```python
from build123d import *

# Parameters (mm, degrees)
SALIENTE_EXTRUIR3_DEPTH = 47
CROQUIS4_W              = 1.5
CROQUIS4_H              = 87
SALIENTE_EXTRUIR4_DEPTH = 47
CROQUIS5_OUTSIDE_W      = 115.342
CROQUIS5_OUTSIDE_H      = 115.342
CROQUIS5_OUTSIDE_R      = 43.5
CORTAR_EXTRUIR1_DEPTH   = 47


with BuildPart() as part:
    # Croquis3 → Saliente-Extruir3 (new body)
    with BuildSketch(Plane(origin=(0, 0, 0), x_dir=(1, 0, 0), z_dir=(0, 1, 0))):
        with BuildLine():
            Line((-43.5, 1.25), (-12.939764295, 1.25))
            ThreePointArc((-12.939764295, 1.25), (0, 13), (12.939764295, 1.25))
            Line((12.939764295, 1.25), (43.5, 1.25))
            Line((43.5, 1.25), (43.5, -1.25))
            Line((43.5, -1.25), (12.939764295, -1.25))
            ThreePointArc((12.939764295, -1.25), (0, -13), (-12.939764295, -1.25))
            Line((-12.939764295, -1.25), (-43.5, -1.25))
            Line((-43.5, -1.25), (-43.5, 1.25))
        make_face()
    extrude(amount=SALIENTE_EXTRUIR3_DEPTH)

    # Croquis4 → Saliente-Extruir4 (add)
    with BuildSketch(Plane(origin=(0, 47, 0), x_dir=(1, 0, 0), z_dir=(0, 1, 0))):
        with Locations((-42.437546, 0)):
            Rectangle(CROQUIS4_W, CROQUIS4_H)
        with Locations((-38.395758095, 0)):
            Rectangle(CROQUIS4_W, CROQUIS4_H)
        with Locations((-34.35397019, 0)):
            Rectangle(CROQUIS4_W, CROQUIS4_H)
        with Locations((-30.312182286, 0)):
            Rectangle(CROQUIS4_W, CROQUIS4_H)
        with Locations((-26.270394381, 0)):
            Rectangle(CROQUIS4_W, CROQUIS4_H)
        with Locations((-22.228606476, 0)):
            Rectangle(CROQUIS4_W, CROQUIS4_H)
        with Locations((-18.186818571, 0)):
            Rectangle(CROQUIS4_W, CROQUIS4_H)
        with Locations((-14.145030667, 0)):
            Rectangle(CROQUIS4_W, CROQUIS4_H)
        with Locations((-10.103242762, 0)):
            Rectangle(CROQUIS4_W, CROQUIS4_H)
        with Locations((-6.061454857, 0)):
            Rectangle(CROQUIS4_W, CROQUIS4_H)
        with Locations((-2.019666952, 0)):
            Rectangle(CROQUIS4_W, CROQUIS4_H)
        with Locations((2.022120952, 0)):
            Rectangle(CROQUIS4_W, CROQUIS4_H)
        with Locations((6.063908857, 0)):
            Rectangle(CROQUIS4_W, CROQUIS4_H)
        with Locations((10.105696762, 0)):
            Rectangle(CROQUIS4_W, CROQUIS4_H)
        with Locations((14.147484667, 0)):
            Rectangle(CROQUIS4_W, CROQUIS4_H)
        with Locations((18.189272571, 0)):
            Rectangle(CROQUIS4_W, CROQUIS4_H)
        with Locations((22.231060476, 0)):
            Rectangle(CROQUIS4_W, CROQUIS4_H)
        with Locations((26.272848381, 0)):
            Rectangle(CROQUIS4_W, CROQUIS4_H)
        with Locations((30.314636286, 0)):
            Rectangle(CROQUIS4_W, CROQUIS4_H)
        with Locations((34.35642419, 0)):
            Rectangle(CROQUIS4_W, CROQUIS4_H)
        with Locations((38.398212095, 0)):
            Rectangle(CROQUIS4_W, CROQUIS4_H)
        with Locations((42.44, 0)):
            Rectangle(CROQUIS4_W, CROQUIS4_H)
    extrude(amount=-SALIENTE_EXTRUIR4_DEPTH)

    # Croquis5 outside → Cortar-Extruir1 (cut)
    with BuildSketch(Plane(origin=(0, 47, 0), x_dir=(1, 0, 0), z_dir=(0, 1, 0))):
        Rectangle(CROQUIS5_OUTSIDE_W, CROQUIS5_OUTSIDE_H)
        Circle(CROQUIS5_OUTSIDE_R, mode=Mode.SUBTRACT)
    extrude(amount=-CORTAR_EXTRUIR1_DEPTH, mode=Mode.SUBTRACT)


solid = part.part
```
Model file for the job. Use its own axes, mm. A direction names the side the tool comes from. Round coordinates to 2 decimals unless told otherwise and drop trailing zeros. Write each loop counter-clockwise with the first axis right and the second up, starting at its lowest first coordinate (ties: lowest second). Pieces come first, ordered by that corner, then holes. Notation, with made-up numbers: (-16.75, 83.5) - (-12.75, 83.5) arc R15 cw to (-12.75, 95.5) - close; hole circle Ø5 at (-27.5, 24.25). An arc over 180 degrees is marked (long way). One line per item, written item: value.
(1) Cut at B-B, the plane x = -20. Give the cut face in (y, z).
Values follow:
outline: (0, -1.25) - (47, -1.25) - (47, 1.25) - (0, 1.25) - close
(2) Wall check: probe 1 along X at (y, z) = (24.5, -0.5); probe 2 along Z at (x, y) = (15.5, 8); probe 3 along Z at (x, y) = (-7, 29.5). Give the ranges that are in metal, low to high.
Values follow:
probe 1: x = -43.5 to 43.5
probe 2: z = -1.25 to 1.25
probe 3: z = -10.95 to 10.95
(3) Drop flat-ended pins along their axis: P1, Ø6, axis at y = 18, z = -13, coming from the -X side (3 decimals); P2, Ø1.3, axis at x = -28, y = 20.5, coming from the +Z side; P3, Ø16.5, axis at y = 31.5, z = 9, coming from the -X side. Give the stop position or say it passes through.
Values follow:
P1: stops at x = -42.335
P2: stops at z = 1.25
P3: stops at x = -43.49
(4) 3-axis set-ups, long thin cutter, end or side, ignore diameter. For faces 1 (the flat face through (-20, 23, -1.25)), 2 (the flat face through (-22.979, 24, 19)): which of +Z, -Z, +X, -X, +Y, -Y reach the whole face in a straight line?
Values follow:
face 1: -Z, +Y, -Y
face 2: +Z, +Y, -Y
(5) Cut at A-A, the plane z = 29. Give the number of separate pieces and of enclosed holes in the cut face, plus the area to 3 significant figures.
Values follow:
separate pieces: 16
enclosed holes: 0
area: 1,130 mm²
